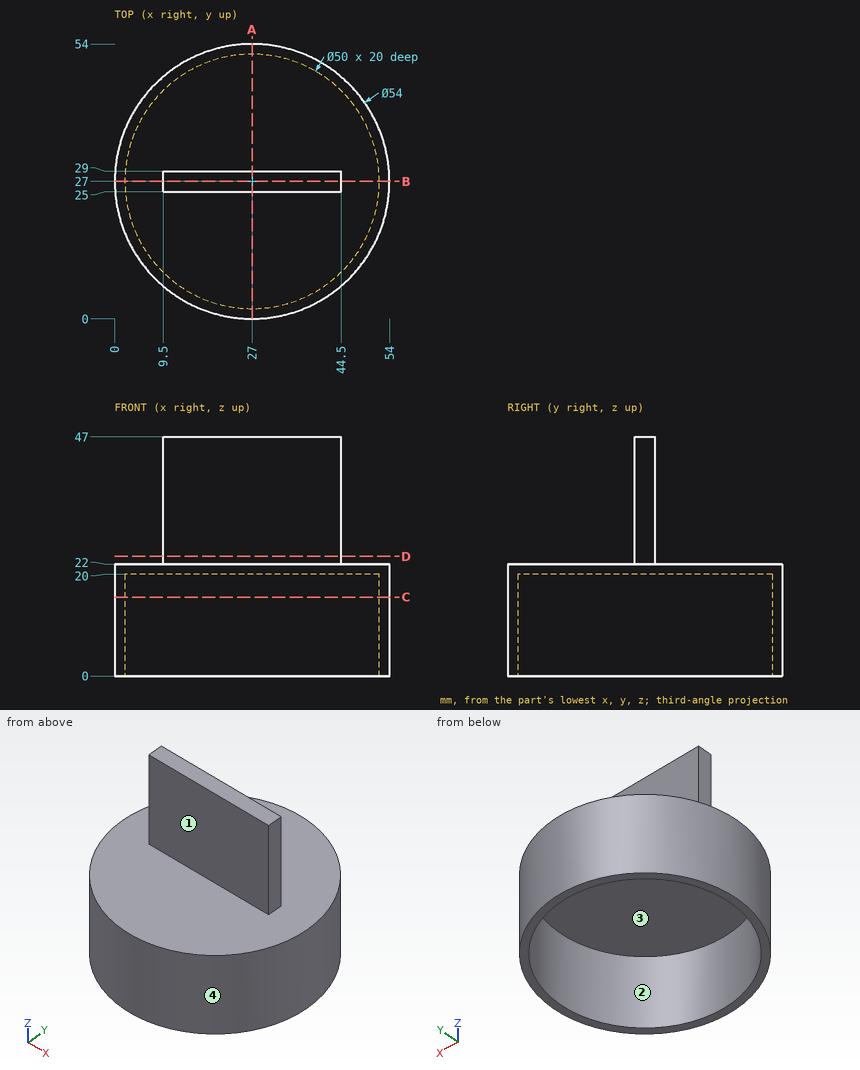
Part print with two shaded views. Sizes in mm from the minimum x, y, z corner. Give positions to 0.01 mm unless a question says otherwise; leave off trailing zeros. Order: outer loops, then holes, each group sorted by start corner. A loop starts at its lowest first (then second) coordinate and runs counter-clockwise, first axis right, second up.
1) Pin check, flat tips, straight feed: pin 1 (12 mm diameter, centred on x = 21, y = 7.5, fed in from +Z); pin 2 (15 mm diameter, centred on x = 23.5, y = 29, fed in from -Z); pin 3 (20 mm diameter, centred on x = 22.5, z = 39, fed in from +Y). Stop position of each tip, or through.
2) Mould opens along Y. For the marked faces 1, 2, 3 and 4 say: +Y half, -Y half, draft (parallel to the pull), parting line (faces both ways), or undercut.
3) Saw through at B-B, the plane y = 27. Write the cut outline in (x, z).
4) Saw through at C-C, the plane z = 15.5. Write the cut outline in (x, y), then the cut area to 3 significant figures.
5) Wall check: probe 1 along Y at (x, z) = (27, 11); probe 2 along Y at (x, z) = (26.5, 33); probe 3 along Z at (x, y) = (24.5, 48). Give the ranges that are in metal, low to high.
6) Saw through at D-D, the plane z = 23.5. Write the cut outline in (x, y).
7) Saw through at A-A, the plane x = 27. Write the cut outline in (y, z), then the cut area to 3 significant figures.
Computed:
1. pin 1: stops at z = 22
1. pin 2: stops at z = 20
1. pin 3: stops at y = 29
2. face 1: -Y half
2. face 2: undercut
2. face 3: undercut
2. face 4: parting line
3. outline: (0, 0) - (2, 0) - (2, 20) - (52, 20) - (52, 0) - (54, 0) - (54, 22) - (44.5, 22) - (44.5, 47) - (9.5, 47) - (9.5, 22) - (0, 22) - close
4. outline: circle Ø54 at (27, 27); hole circle Ø50 at (27, 27)
4. area: 327 mm2
5. probe 1: y = 0 to 2, 52 to 54
5. probe 2: y = 25 to 29
5. probe 3: z = 20 to 22
6. outline: (9.5, 25) - (44.5, 25) - (44.5, 29) - (9.5, 29) - close
7. outline: (0, 0) - (2, 0) - (2, 20) - (52, 20) - (52, 0) - (54, 0) - (54, 22) - (29, 22) - (29, 47) - (25, 47) - (25, 22) - (0, 22) - close
7. area: 288 mm2
